from build123d import *

# Parameters (mm, degrees)
SKETCH1_R           = 7.5
BOSS_EXTRUDE1_DEPTH = 2
SKETCH2_R           = 1.5
BOSS_EXTRUDE2_DEPTH = 15


with BuildPart() as part:
    # Sketch1 → Boss-Extrude1 (new body)
    with BuildSketch(Plane(origin=(0, 0, 0), x_dir=(1, 0, 0), z_dir=(0, 1, 0))):
        Circle(SKETCH1_R)
    extrude(amount=BOSS_EXTRUDE1_DEPTH)

    # Sketch2 → Boss-Extrude2 (add)
    with BuildSketch(Plane(origin=(0, 2, 0), x_dir=(1, 0, 0), z_dir=(0, 1, 0))):
        with Locations((0.294077072, -4.75)):
            Circle(SKETCH2_R)
        with Locations((0.294077072, 4.75)):
            Circle(SKETCH2_R)
        with Locations((4.294077072, 0)):
            Circle(SKETCH2_R)
    extrude(amount=BOSS_EXTRUDE2_DEPTH)


solid = part.part
Verification items for the finished model (mm, model axes). A direction names the side the tool comes from. Coordinates: 2 decimals unless noted, no trailing zeros. Order: outer loops, then holes, each group sorted by start corner. A loop starts at its lowest first (then second) coordinate and runs counter-clockwise, first axis right, second up. Notation, with made-up numbers: M -22.75,85 L 24.25,85 A34 cw 24.25,123 Z; hole C -28.5,66 d8. An arc over 180 degrees is marked long. Return JSON: item names as keys, results as strings.
1) Access from +Z, -Z, +X, -X, +Y, -Y to the whole of each face (thin tool, end or side, straight path). Record for faces 1 (the flat face through (0, 17, -5)), 2 (the cylindrical face through (-1.204, 9.395, -4.816)).
Answer list:
{"face 1": "+Z, -Z, +X, -X, +Y", "face 2": "+Y"}
2) Cross-section at C-C, the plane x = 0. Record the boundary of the cut face in (y, z).
Answer list:
{"outline": "M 0,-7.5 L 2,-7.5 L 2,-6.22 L 17,-6.22 L 17,-3.28 L 2,-3.28 L 2,3.28 L 17,3.28 L 17,6.22 L 2,6.22 L 2,7.5 L 0,7.5 Z"}
3) Gauge pin test, flat ends, axial feed: pin 1 (1.5 mm diameter, centred on x = -1, y = 2, fed in from -Z); pin 2 (8 mm diameter, centred on y = 14, z = 2.5, fed in from +X); pin 3 (6 mm diameter, centred on y = 3, z = 3, fed in from +X). Record the tip position at first contact, or that the pin passes through.
Answer list:
{"pin 1": "z = -7.5", "pin 2": "x = 5.79", "pin 3": "x = 7.5"}
4) Cross-section at B-B, the plane z = 0. Record the boundary of the cut face in (x, y).
Answer list:
{"outline": "M -7.5,0 L 7.5,0 L 7.5,2 L 5.79,2 L 5.79,17 L 2.79,17 L 2.79,2 L -7.5,2 Z"}
5) Cross-section at D-D, the plane z = 6. Record the boundary of the cut face in (x, y), and give its area (3 significant figures).
Answer list:
{"outline": "M -4.5,0 L 4.5,0 L 4.5,2 L 1.12,2 L 1.12,17 L -0.54,17 L -0.54,2 L -4.5,2 Z", "area": "42.9 mm2"}
6) Cross-section at A-A, the plane y = 14.75. Record the boundary of the cut face in (x, z), and give its area (3 significant figures).
Answer list:
{"outline": "C 0.29,-4.75 d3; C 0.29,4.75 d3; C 4.29,0 d3", "area": "21.2 mm2"}
7) Thickness scan on L1, parallel to Y at x = -0.75, z = 0.5; L2, parallel to Z at x = 0.5, y = 15.5; L3, parallel to X at y = 16.75, z = -3.75. Record the ranges inside material, lowest first. Write a range as [from, to].
Answer list:
{"L1": "[0, 2]", "L2": "[-6.24, -3.26], [3.26, 6.24]", "L3": "[-0.82, 1.41]"}
